Verification items for this drawing (mm, ordinates from the low corner). Give positions to 0.01 mm unless a question says otherwise; leave off trailing zeros. Order: outer loops, then holes, each group sorted by start corner. A loop starts at its lowest first (then second) coordinate and runs counter-clockwise, first axis right, second up. Notation, with made-up numbers: M 68.5,-13 L 127.5,-13 A22 cw 127.5,-1 Z; hole C 73.5,-15.5 d6. An arc over 180 degrees is marked long. Answer as a JSON object with one key per item and string values.
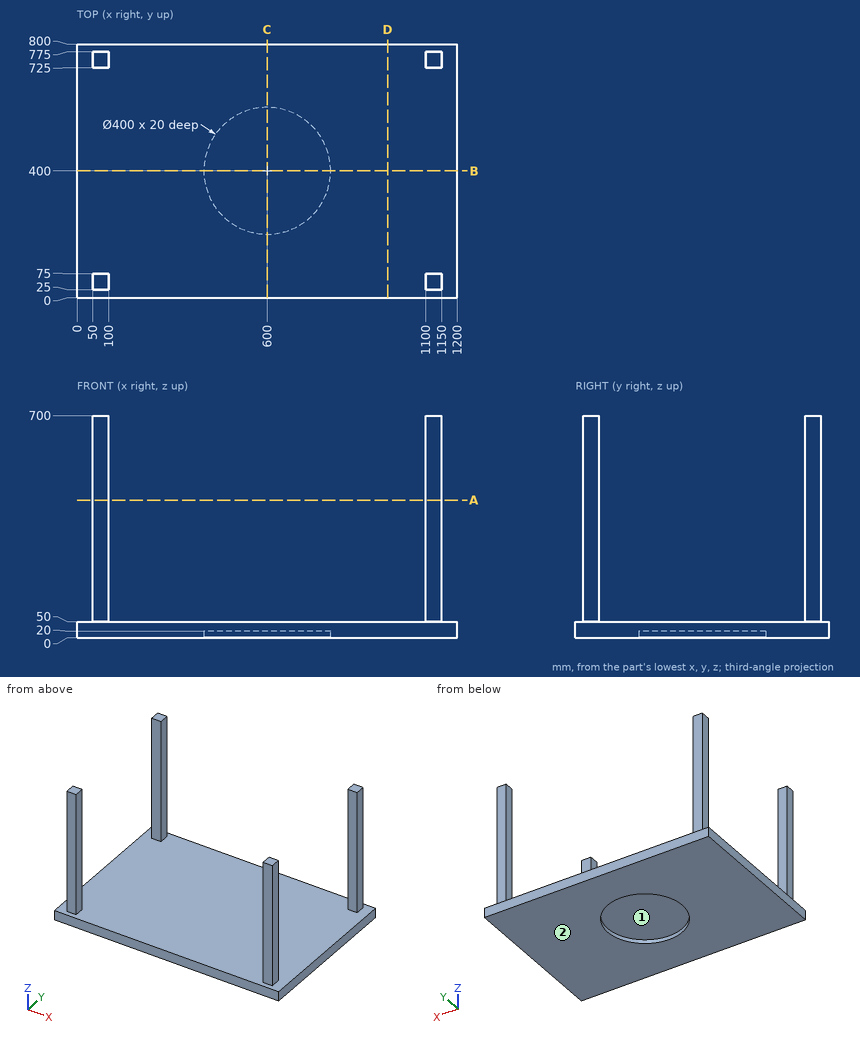
Q1. Section check D-D on x = 980. Record the cut outline in (y, z), then the cut area to 3 significant figures.
Resolved:
{"outline": "M 0,0 L 800,0 L 800,50 L 0,50 Z", "area": "40,000 mm²"}
Q2. Section check C-C on x = 600. Record the cut outline in (y, z).
Resolved:
{"outline": "M 0,0 L 200,0 L 200,20 L 600,20 L 600,0 L 800,0 L 800,50 L 0,50 Z"}
Q3. Section check B-B on y = 400. Record the cut outline in (x, z).
Resolved:
{"outline": "M 0,0 L 400,0 L 400,20 L 800,20 L 800,0 L 1200,0 L 1200,50 L 0,50 Z"}
Q4. Gauge pin test, flat ends, axial feed: pin 1 Ø3 at (x, y) = (1063.5, 560) entering from +Z; pin 2 Ø15 at (y, z) = (743, 348.5) entering from -X; pin 3 Ø4 at (x, y) = (688.5, 387.5) entering from -Z. Record the tip position at first contact, or that the pin passes through.
Resolved:
{"pin 1": "stops at z = 50", "pin 2": "stops at x = 50", "pin 3": "stops at z = 20"}
Q5. Release check for a two-part mould opening along X. For the marked faces 1 and 2 record: +X half, -X half, draft (parallel to the pull), parting line (faces both ways), or undercut.
Resolved:
{"face 1": "undercut", "face 2": "draft"}
Q6. Section check A-A on z = 433. Record the cut outline in (x, y), then the cut area to 3 significant figures.
Resolved:
{"outline": "M 50,25 L 100,25 L 100,75 L 50,75 Z; M 50,725 L 100,725 L 100,775 L 50,775 Z; M 1100,25 L 1150,25 L 1150,75 L 1100,75 Z; M 1100,725 L 1150,725 L 1150,775 L 1100,775 Z", "area": "10,000 mm²"}
Q7. Material ranges on L1, parallel to Y at x = 600, z = 9; L2, parallel to X at y = 57, z = 470; L3, parallel to Z at x = 270, y = 567, recorded low to high.
Resolved:
{"L1": "y = 0 to 200, 600 to 800", "L2": "x = 50 to 100, 1100 to 1150", "L3": "z = 0 to 50"}
